from build123d import *

# Parameters (mm, degrees)
SKETCH1_R                         = 12.7
BOSS_EXTRUDE1_DEPTH               = 79.375
SKETCH2_R                         = 21.293421543
SKETCH2_R_2                       = 9.525
CUT_EXTRUDE1_DEPTH                = 19.05
SKETCH3_W                         = 88.347660667
SKETCH3_H                         = 62.084650607
CUT_EXTRUDE2_DEPTH                = 7.62
SKETCH7_W                         = 118.824828897
SKETCH7_H                         = 51.847980611
CUT_EXTRUDE5_DEPTH                = 25.4
F_1_4_20_TAPPED_HOLE2_D           = 5.1054
F_1_4_20_TAPPED_HOLE2_DEPTH       = 16.002
F_1_4_20_TAPPED_HOLE2_CSINK_D     = 7.112
F_1_4_20_TAPPED_HOLE2_CSINK_ANGLE = 82
F_1_4_20_TAPPED_HOLE2_TIP         = 1.533816902
F_1_4_20_TAPPED_HOLE3_D           = 5.1054
F_1_4_20_TAPPED_HOLE3_DEPTH       = 16.002
F_1_4_20_TAPPED_HOLE3_CSINK_D     = 7.112
F_1_4_20_TAPPED_HOLE3_CSINK_ANGLE = 82
F_1_4_20_TAPPED_HOLE3_TIP         = 1.533816902


with BuildPart() as part:
    # Sketch1 → Boss-Extrude1 (new body)
    with BuildSketch(Plane(origin=(0, 0, 0), x_dir=(0, 0, -1), z_dir=(1, 0, 0))):
        Circle(SKETCH1_R)
    extrude(amount=-BOSS_EXTRUDE1_DEPTH)

    # Sketch2 → Cut-Extrude1 (cut)
    with BuildSketch(Plane(origin=(0, 0, 0), x_dir=(0, 0, -1), z_dir=(1, 0, 0))):
        Circle(SKETCH2_R)
        Circle(SKETCH2_R_2, mode=Mode.SUBTRACT)
    extrude(amount=-CUT_EXTRUDE1_DEPTH, mode=Mode.SUBTRACT)

    # Sketch3 → Cut-Extrude2 (cut)
    with BuildSketch(Plane(origin=(0, 12.401228443, 11.1252), x_dir=(1, 0, 0), z_dir=(0, 0, 1))):
        with Locations((-47.069787049, -6.880973923)):
            Rectangle(SKETCH3_W, SKETCH3_H)
    extrude(amount=CUT_EXTRUDE2_DEPTH, mode=Mode.SUBTRACT)

    # Sketch7 → Cut-Extrude5 (cut)
    with BuildSketch(Plane(origin=(0, 11.1252, 0), x_dir=(-1, 0, 0), z_dir=(0, 1, 0))):
        with Locations((37.000899043, -1.114295637)):
            Rectangle(SKETCH7_W, SKETCH7_H)
    extrude(amount=CUT_EXTRUDE5_DEPTH, mode=Mode.SUBTRACT)

    # 1/4-20 Tapped Hole2
    with Locations(Plane(origin=(0, 11.1252, 0), x_dir=(-1, 0, 0), z_dir=(0, 1, 0))):
        with Locations((25.4, 0)):
            CounterSinkHole(F_1_4_20_TAPPED_HOLE2_D / 2, F_1_4_20_TAPPED_HOLE2_CSINK_D / 2, depth=F_1_4_20_TAPPED_HOLE2_DEPTH, counter_sink_angle=F_1_4_20_TAPPED_HOLE2_CSINK_ANGLE)
            with Locations((0, 0, -(F_1_4_20_TAPPED_HOLE2_DEPTH + F_1_4_20_TAPPED_HOLE2_TIP / 2))):  # 118° drill point
                Cone(0, F_1_4_20_TAPPED_HOLE2_D / 2, F_1_4_20_TAPPED_HOLE2_TIP, mode=Mode.SUBTRACT)

    # 1/4-20 Tapped Hole3
    with Locations(Plane(origin=(0, 0, 0), x_dir=(0, 0, -1), z_dir=(1, 0, 0))):
        with Locations((0, 0)):
            CounterSinkHole(F_1_4_20_TAPPED_HOLE3_D / 2, F_1_4_20_TAPPED_HOLE3_CSINK_D / 2, depth=F_1_4_20_TAPPED_HOLE3_DEPTH, counter_sink_angle=F_1_4_20_TAPPED_HOLE3_CSINK_ANGLE)
            with Locations((0, 0, -(F_1_4_20_TAPPED_HOLE3_DEPTH + F_1_4_20_TAPPED_HOLE3_TIP / 2))):  # 118° drill point
                Cone(0, F_1_4_20_TAPPED_HOLE3_D / 2, F_1_4_20_TAPPED_HOLE3_TIP, mode=Mode.SUBTRACT)


solid = part.part
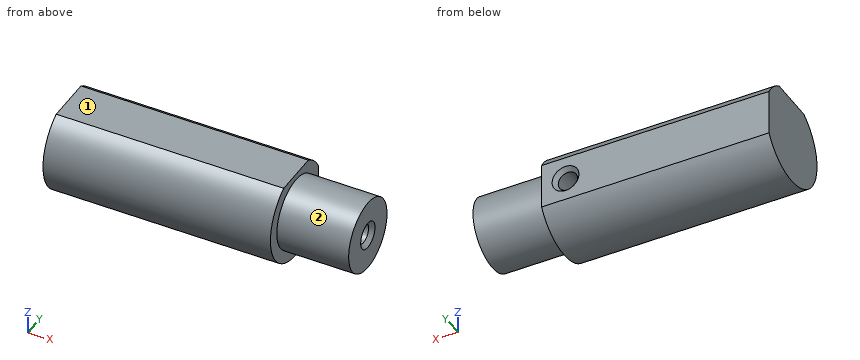
Read the model definition and answer for the solid it produces. Units are mm, in the model's axes. Face numbers are marked on the shaded views. A direction names the side the tool comes from. Coordinates: 2 decimals unless noted, no trailing zeros. Loops run counter-clockwise (first coordinate to the right, second up) from the corner with the lowest first, then second, coordinate; pieces in that order, holes last. Notation, with made-up numbers: (85.25, -35) -> (106.25, -35) arc R26 cw to (106.25, -19) -> close; hole circle Ø8 at (-16, -38). An arc over 180 degrees is marked (long way). Write item = value, one per line. Start each with the question number.
1) Given P1, Ø10, axis at x = -19.5, z = -3.5, coming from the -Y side; P2, Ø1, axis at y = 7.5, z = 7.5, coming from the +X side; P3, Ø5, axis at x = -9.5, z = 6, coming from the +Y side; P4, Ø3, axis at x = -36, y = 7.5, coming from the -Z side, each flat-ended and moving along its own axis, determine where each tip first touches the part or whether it passes through.
2) The part is cut by section A-A, the plane x = -14. Determine the outline of the cut face in (y, z) (3 decimals).
3) The part is cut by section D-D, the plane x = -43.5. Determine the outline of the cut face in (y, z), plus the area to 3 significant figures.
4) For the marked faces 1 and 2, determine the directions among +Z, -Z, +X, -X, +Y, -Y from which every point of the face is accessible in a straight line to the end or side of a thin tool.
5) Find the intervals of material crossed by L1, parallel to X at y = 4.5, z = 0 (3 decimals); L2, parallel to X at y = 0, z = 0 (3 decimals); L3, parallel to Y at x = -4.75, z = 0 (3 decimals), in increasing order. Write a range as from..to.
6) The part is cut by section C-C, the plane z = 7.5. Determine the outline of the cut face in (x, y) (3 decimals).
7) The part is cut by section B-B, the plane y = 7.25. Determine the outline of the cut face in (x, z) (3 decimals), plus the area to 3 significant figures.
Result:
q1.P1 = -12.7
q1.P2 = -19.05
q1.P3 = 8.86
q1.P4 = -11.19
q2.outline = circle Ø19.05 at (0, 0); hole circle Ø5.105 at (0, 0)
q3.outline = (-6.13, 11.13) arc R12.7 ccw (long way) to (11.13, -6.13) -> (11.13, 6.13) arc R12.7 ccw to (6.13, 11.13) -> close
q3.area = 481 mm²
q4.face_1 = +Z, +X, -X, +Y, -Y
q4.face_2 = +X
q5.L1 = -79.375..-27.953, -22.847..0
q5.L2 = -79.375..-27.953, -22.847..-17.536
q5.L3 = -9.525..-2.553, 2.553..9.525
q6.outline = (-79.375, -10.249) -> (-19.05, -10.249) -> (-19.05, -5.872) -> (0, -5.872) -> (0, 5.872) -> (-19.05, 5.872) -> (-19.05, 10.249) -> (-79.375, 10.249) -> close
q7.outline = (-79.375, -10.427) -> (-19.05, -10.427) -> (-19.05, -6.178) -> (0, -6.178) -> (0, 6.178) -> (-19.05, 6.178) -> (-19.05, 10.427) -> (-79.375, 10.427) -> close; hole circle Ø5.105 at (-25.4, 0)
q7.area = 1,470 mm²
